from build123d import *

# Parameters (mm, degrees)
SKETCH1_R                                        = 40
BOSS_EXTRUDE1_DEPTH                              = 10
CBORE_FOR_M6_HEX_HEAD_MACHINE_SCREW1_D           = 6.6
CBORE_FOR_M6_HEX_HEAD_MACHINE_SCREW1_CBORE_D     = 13.95
CBORE_FOR_M6_HEX_HEAD_MACHINE_SCREW1_CBORE_DEPTH = 4.7
M4_CLEARANCE_HOLE1_D                             = 4.5
SKETCH6_R                                        = 8.5
CUT_EXTRUDE1_DEPTH                               = 2


with BuildPart() as part:
    # Sketch1 → Boss-Extrude1 (new body)
    with BuildSketch(Plane.XY):
        Circle(SKETCH1_R)
    extrude(amount=BOSS_EXTRUDE1_DEPTH)

    # CBORE for M6 Hex Head Machine Screw1 (through all)
    with Locations(Plane.XY.offset(10)):
        with Locations((0, 0)):
            CounterBoreHole(CBORE_FOR_M6_HEX_HEAD_MACHINE_SCREW1_D / 2, CBORE_FOR_M6_HEX_HEAD_MACHINE_SCREW1_CBORE_D / 2, CBORE_FOR_M6_HEX_HEAD_MACHINE_SCREW1_CBORE_DEPTH)

    # M4 Clearance Hole1 (through all)
    with Locations(Plane.XY.offset(10)):
        with Locations((0, 32), (32, 0), (0, -32), (-32, 0)):
            Hole(M4_CLEARANCE_HOLE1_D / 2)

    # Sketch6 → Cut-Extrude1 (cut)
    with BuildSketch(Plane(origin=(0, 0, 0), x_dir=(-1, 0, 0), z_dir=(0, 0, -1))):
        Circle(SKETCH6_R)
    extrude(amount=-CUT_EXTRUDE1_DEPTH, mode=Mode.SUBTRACT)


solid = part.part
Read the model definition and answer for the solid it produces. Units are mm, in the model's axes. A direction names the side the tool comes from. Give positions to 0.01 mm unless a question says otherwise; leave off trailing zeros. Loops run counter-clockwise (first coordinate to the right, second up) from the corner with the lowest first, then second, coordinate; pieces in that order, holes last. Notation, with made-up numbers: M 8,-21 L 24,-21 A27 ccw 24,2 Z; hole C -23.75,39.5 d2. An arc over 180 degrees is marked long. Write each question's results on one line, items separated by ' | '.
1. Section B-B on z = 8.75 is taken. Give the vertices of the cut face in (x, y) (3 decimals), plus the area to 3 significant figures.
Values:
outline: C 0,0 d80; hole C -32,0 d4.5; hole C 0,0 d13.95; hole C 0,-32 d4.5; hole C 0,32 d4.5; hole C 32,0 d4.5 | area: 4,810 mm^2
2. Section A-A on y = 32 is taken. Give the vertices of the cut face in (x, z).
Values:
outline: M -24,0 L -2.25,0 L -2.25,10 L -24,10 Z; M 2.25,0 L 24,0 L 24,10 L 2.25,10 Z
3. Section D-D on z = 3.75 is taken. Give the vertices of the cut face in (x, y).
Values:
outline: C 0,0 d80; hole C -32,0 d4.5; hole C 0,0 d6.6; hole C 0,-32 d4.5; hole C 0,32 d4.5; hole C 32,0 d4.5
4. A tool of negligible diameter and unlimited length cuts with its end or side. For faces 1 (the face through (-4, 0, 2)), 2 (the face through (-1.51, -6.81, 7.68)), 3 (the face through (2.43, 2.23, 3.63)), from which of +Z, -Z, +X, -X, +Y, -Y can it reach the whole face along a straight path? Write none if from no direction.
Values:
face 1: -Z | face 2: +Z | face 3: +Z, -Z
5. Straight lines are drawn through the part: line 1 (Y direction, x = 0, z = 3.65); line 2 (Y direction, x = -32, z = 2.5); line 3 (Y direction, x = 31.5, z = 8). For each, find the intervals that lie inside material, in ascending order. Write a range as [from, to].
Values:
line 1: y = [-40, -34.25], [-29.75, -3.3], [3.3, 29.75], [34.25, 40] | line 2: y = [-24, -2.25], [2.25, 24] | line 3: y = [-24.65, -2.19], [2.19, 24.65]
6. The mould has two halves that part along X. Classify faces 4 (the face through (-1, 9, 0)), 5 (the face through (-8.67, -39.05, 4.93)), 6 (the face through (3, 2, 5.3)): pulls with the +X half, pulls with the -X half, needs draft (parallel to the pull), parting line crosses it, or undercut.
Values:
face 4: needs draft | face 5: parting line crosses it | face 6: undercut
7. Given pin 1 (1 mm diameter, centred on y = -6, z = 3, fed in from +X); pin 2 (4 mm diameter, centred on x = 24.5, z = 4.5, fed in from +Y); pin 3 (1.5 mm diameter, centred on y = 5.5, z = 5, fed in from +X); pin 4 (3.5 mm diameter, centred on x = 0, y = 32, fed in from +Z), each flat-ended and moving along its own axis, determine where each tip first touches the part or whether it passes through.
Values:
pin 1: stops at x = 39.62 | pin 2: stops at y = 33.07 | pin 3: stops at x = 39.72 | pin 4: passes through
